```python
from build123d import *

# Parameters (mm, degrees)
ESBO_O1_W                 = 20
ESBO_O1_H                 = 30
RESSALTO_EXTRUS_O1_DEPTH  = 2.5
ESBO_O2_W                 = 5.5
ESBO_O2_H                 = 16
CORTE_EXTRUS_O1_DEPTH     = 5
FILETE1_R                 = 1
FILETE2_R                 = 2
FILETE3_R                 = 2
FILETE4_R                 = 1
FILETE5_R                 = 1
FILETE6_R                 = 1
ESBO_O3_W                 = 1.2
ESBO_O3_H                 = 20
CORTE_EXTRUS_O2_DEPTH     = 1
CHANFRO1_SIZE             = 0.5
CHANFRO3_SIZE             = 0.5
FILETE1_OF_ESPELHAR6_R    = 1
ESPELHAR7_COPY_1_SKETCH_W = 1.2
ESPELHAR7_COPY_1_SKETCH_H = 20
ESPELHAR7_COPY_1_DEPTH    = 1
ESPELHAR7_COPY_2_SKETCH_W = 1.2
ESPELHAR7_COPY_2_SKETCH_H = 20
ESPELHAR7_COPY_2_DEPTH    = 1
FILETE7_R                 = 2
FILETE8_R                 = 2
FILETE9_R                 = 1
CHANFRO4_SIZE             = 0.5
CHANFRO5_SIZE             = 0.5
FILETE10_R                = 1
FILETE11_R                = 1


with BuildPart() as part:
    # Esboço1 → Ressalto-extrusão1 (new body)
    with BuildSketch(Plane(origin=(0, 0, 0), x_dir=(1, 0, 0), z_dir=(0, 1, 0))):
        Rectangle(ESBO_O1_W, ESBO_O1_H)
    ressalto_extrus_o1 = extrude(amount=RESSALTO_EXTRUS_O1_DEPTH)

    # Esboço2 → Corte-extrusão1 (cut)
    with BuildSketch(Plane(origin=(0, 2.5, 0), x_dir=(1, 0, 0), z_dir=(0, 1, 0))):
        with Locations((0, -7)):
            Rectangle(ESBO_O2_W, ESBO_O2_H)
    corte_extrus_o1 = extrude(amount=-CORTE_EXTRUS_O1_DEPTH, mode=Mode.SUBTRACT)

    # Filete1
    filete1_edges = [part.edges().sort_by_distance(p)[0] for p in [
        (10, 1.25, 15),
    ]]
    fillet(filete1_edges, radius=FILETE1_R)

    # Filete2
    filete2_edges = [part.edges().sort_by_distance(p)[0] for p in [
        (10, 1.25, -15),
    ]]
    fillet(filete2_edges, radius=FILETE2_R)

    # Filete3
    filete3_edges = [part.edges().sort_by_distance(p)[0] for p in [
        (-10, 1.25, -15),
    ]]
    fillet(filete3_edges, radius=FILETE3_R)

    # Filete4
    filete4_edges = [part.edges().sort_by_distance(p)[0] for p in [
        (-10, 1.25, 15),
    ]]
    fillet(filete4_edges, radius=FILETE4_R)

    # Filete5
    filete5_edges = [part.edges().sort_by_distance(p)[0] for p in [
        (-2.75, 1.25, 15),
    ]]
    fillet(filete5_edges, radius=FILETE5_R)

    # Filete6
    filete6_edges = [part.edges().sort_by_distance(p)[0] for p in [
        (2.75, 1.25, 15),
    ]]
    fillet(filete6_edges, radius=FILETE6_R)

    # Esboço3 → Corte-extrusão2 (cut)
    with BuildSketch(Plane(origin=(0, 2.5, 0), x_dir=(1, 0, 0), z_dir=(0, 1, 0))):
        with Locations((-4.475, -5)):
            Rectangle(ESBO_O3_W, ESBO_O3_H)
        with Locations((-6.475, -5)):
            Rectangle(ESBO_O3_W, ESBO_O3_H)
        with Locations((-8.475, -5)):
            Rectangle(ESBO_O3_W, ESBO_O3_H)
    corte_extrus_o2 = extrude(amount=-CORTE_EXTRUS_O2_DEPTH, mode=Mode.SUBTRACT)

    # Chanfro1
    chanfro1_edges = [part.edges().sort_by_distance(p)[0] for p in [
        (-7.875, 1.5, 5),
        (-9.075, 1.5, 4.998591767),
        (-3.875, 1.5, 5),
        (-4.475, 1.5, -5),
        (-5.075, 1.5, 5),
        (-5.875, 1.5, 5),
        (-6.475, 1.5, -5),
        (-7.075, 1.5, 5),
        (-8.475, 1.5, -5),
    ]]
    chamfer(chanfro1_edges, length=CHANFRO1_SIZE)

    # Espelhar4: Corte-extrusão2 across plane
    add(corte_extrus_o2.mirror(Plane(origin=(0, 0, 0), x_dir=(0, 0, 1), z_dir=(1, 0, 0))), mode=Mode.SUBTRACT)

    # Chanfro3
    chanfro3_edges = [part.edges().sort_by_distance(p)[0] for p in [
        (9.075, 1.5, 4.998591767),
        (8.475, 1.5, -5),
        (7.875, 1.5, 5),
        (7.075, 1.5, 5),
        (6.475, 1.5, -5),
        (5.875, 1.5, 5),
        (5.075, 1.5, 5),
        (4.475, 1.5, -5),
        (3.875, 1.5, 5),
    ]]
    chamfer(chanfro3_edges, length=CHANFRO3_SIZE)

    # Espelhar5: Ressalto-extrusão1 across plane
    add(ressalto_extrus_o1.mirror(Plane.ZX))

    # Espelhar6: Corte-extrusão2 across plane
    add(corte_extrus_o2.mirror(Plane.ZX), mode=Mode.SUBTRACT)

    # Filete1 of Espelhar6
    filete1_of_espelhar6_edges = [part.edges().sort_by_distance(p)[0] for p in [
        (10, -1.25, 15),
    ]]
    fillet(filete1_of_espelhar6_edges, radius=FILETE1_OF_ESPELHAR6_R)

    # Espelhar7 copy 1 sketch → Espelhar7 copy 1 (cut)
    with BuildSketch(Plane(origin=(0, -2.5, 0), x_dir=(-1, 0, 0), z_dir=(0, -1, 0))):
        with Locations((-4.475, -5)):
            Rectangle(ESPELHAR7_COPY_1_SKETCH_W, ESPELHAR7_COPY_1_SKETCH_H)
        with Locations((-6.475, -5)):
            Rectangle(ESPELHAR7_COPY_1_SKETCH_W, ESPELHAR7_COPY_1_SKETCH_H)
        with Locations((-8.475, -5)):
            Rectangle(ESPELHAR7_COPY_1_SKETCH_W, ESPELHAR7_COPY_1_SKETCH_H)
    extrude(amount=-ESPELHAR7_COPY_1_DEPTH, mode=Mode.SUBTRACT)

    # Espelhar7 copy 2 sketch → Espelhar7 copy 2 (cut)
    with BuildSketch(Plane.XZ.offset(2.5)):
        with Locations((-4.475, 5)):
            Rectangle(ESPELHAR7_COPY_2_SKETCH_W, ESPELHAR7_COPY_2_SKETCH_H)
        with Locations((-6.475, 5)):
            Rectangle(ESPELHAR7_COPY_2_SKETCH_W, ESPELHAR7_COPY_2_SKETCH_H)
        with Locations((-8.475, 5)):
            Rectangle(ESPELHAR7_COPY_2_SKETCH_W, ESPELHAR7_COPY_2_SKETCH_H)
    extrude(amount=-ESPELHAR7_COPY_2_DEPTH, mode=Mode.SUBTRACT)

    # Filete7
    filete7_edges = [part.edges().sort_by_distance(p)[0] for p in [
        (10, -1.25, -15),
    ]]
    fillet(filete7_edges, radius=FILETE7_R)

    # Filete8
    filete8_edges = [part.edges().sort_by_distance(p)[0] for p in [
        (-10, -1.25, -15),
    ]]
    fillet(filete8_edges, radius=FILETE8_R)

    # Filete9
    filete9_edges = [part.edges().sort_by_distance(p)[0] for p in [
        (-10, -1.25, 15),
    ]]
    fillet(filete9_edges, radius=FILETE9_R)

    # Chanfro4
    chanfro4_edges = [part.edges().sort_by_distance(p)[0] for p in [
        (3.875, -1.5, 5),
        (4.475, -1.5, -5),
        (5.075, -1.5, 5),
        (5.875, -1.5, 5),
        (6.475, -1.5, -5),
        (7.075, -1.5, 5),
        (7.875, -1.5, 5),
        (8.475, -1.5, -5),
        (9.075, -1.5, 4.998591767),
    ]]
    chamfer(chanfro4_edges, length=CHANFRO4_SIZE)

    # Chanfro5
    chanfro5_edges = [part.edges().sort_by_distance(p)[0] for p in [
        (-9.075, -1.5, 4.998591767),
        (-8.475, -1.5, -5),
        (-7.875, -1.5, 5),
        (-7.075, -1.5, 5),
        (-6.475, -1.5, -5),
        (-5.875, -1.5, 5),
        (-5.075, -1.5, 5),
        (-4.475, -1.5, -5),
        (-3.875, -1.5, 5),
    ]]
    chamfer(chanfro5_edges, length=CHANFRO5_SIZE)

    # Espelhar8: Corte-extrusão1 across plane
    add(corte_extrus_o1.mirror(Plane.ZX), mode=Mode.SUBTRACT)

    # Filete10
    filete10_edges = [part.edges().sort_by_distance(p)[0] for p in [
        (2.75, -1.25, 15),
    ]]
    fillet(filete10_edges, radius=FILETE10_R)

    # Filete11
    filete11_edges = [part.edges().sort_by_distance(p)[0] for p in [
        (-2.75, -1.25, 15),
    ]]
    fillet(filete11_edges, radius=FILETE11_R)


solid = part.part
```
For this review, take the finished solid that the model builds, in its own axes (mm). A direction names the side the tool comes from. Coordinates: 2 decimals unless noted, no trailing zeros. Write each loop counter-clockwise with the first axis right and the second up, starting at its lowest first coordinate (ties: lowest second). Pieces come first, ordered by that corner, then holes. Notation, with made-up numbers: (-9.5, 47) - (4.5, 47) arc R32 cw to (4.5, 84) - close; hole circle Ø9 at (-12, -11). An arc over 180 degrees is marked (long way). Answer in a Markdown table with one row per item. Add a question column.
Q1. For P1, Ø4, axis at x = 1.5, z = 3.5, coming from the +Y side; P2, Ø0.6, axis at x = 6.5, y = -2.5, coming from the +Z side, all flat-tipped, find the tip position at first contact; note any pin that passes through.
Q2. For probe 1 along X at (y, z) = (-1.4, 11); probe 2 along Z at (x, y) = (-2.25, 1.75); probe 3 along Z at (x, y) = (-4, -2.3), list the stretches that pass through material, from the lowest coordinate up.
Q3. Tool access review of faces 1 (the flat face through (-3, 0, 15)), 2 (the flat face through (-10, 0, 1)): name each direction out of +Z, -Z, +X, -X, +Y, -Y from which nothing blocks a thin tool from reaching the whole face with its end or side.
Q4. Draft analysis for pull direction X (two halves, no side actions). For faces 3 (the cylindrical face through (3.035, -1.232, 14.699)), 4 (the flat face through (2.75, 0, 7)), 5 (the cylindrical face through (9.4, -1.27, -14.43)), 6 (the flat face through (0, 0, -15)), state which applies: +X half, -X half, draft (parallel to the pull), parting line (faces both ways), or undercut.
Q5. We need section A-A, the plane y = 0.3. State the section outline as (x, z) points, and give its area (3 significant figures).
Answer list:
| question | item | result |
|---|---|---|
| 1 | P1 | stops at y = 2.5 |
| 1 | P2 | stops at z = -5 |
| 2 | probe 1 | x = -10 to -2.75, 2.75 to 10 |
| 2 | probe 2 | z = -15 to -1 |
| 2 | probe 3 | z = -15 to -5 |
| 3 | face 1 | none |
| 3 | face 2 | +Z, -Z, -X, +Y, -Y |
| 4 | face 3 | undercut |
| 4 | face 4 | undercut |
| 4 | face 5 | +X half |
| 4 | face 6 | draft |
| 5 | outline | (-10, -13) arc R2 ccw to (-8, -15) - (8, -15) arc R2 ccw to (10, -13) - (10, 14) arc R1 ccw to (9, 15) - (3.75, 15) arc R1 ccw to (2.75, 14) - (2.75, -1) - (-2.75, -1) - (-2.75, 14) arc R1 ccw to (-3.75, 15) - (-9, 15) arc R1 ccw to (-10, 14) - close |
| 5 | area | 509 mm2 |
